from build123d import *

# Parameters (mm, degrees)
SKETCH1_W           = 40
SKETCH1_H           = 8
SKETCH1_R           = 0.75
BOSS_EXTRUDE1_DEPTH = 3
SKETCH2_W           = 19
SKETCH2_H           = 8
BOSS_EXTRUDE2_DEPTH = 15
SKETCH3_W           = 12.3
SKETCH3_H           = 29.8
CUT_EXTRUDE1_DEPTH  = 8
FILLET1_R           = 1


with BuildPart() as part:
    # Sketch1 → Boss-Extrude1 (new body)
    with BuildSketch(Plane.XY):
        Rectangle(SKETCH1_W, SKETCH1_H)
        with Locations((-14.5, 0)):
            Circle(SKETCH1_R, mode=Mode.SUBTRACT)
        with Locations((14.5, 0)):
            Circle(SKETCH1_R, mode=Mode.SUBTRACT)
    extrude(amount=BOSS_EXTRUDE1_DEPTH)

    # Sketch2 → Boss-Extrude2 (add)
    with BuildSketch(Plane.XY.offset(3)):
        Rectangle(SKETCH2_W, SKETCH2_H)
    extrude(amount=BOSS_EXTRUDE2_DEPTH)

    # Sketch3 → Cut-Extrude1 (cut)
    with BuildSketch(Plane.XZ.offset(4)):
        Rectangle(SKETCH3_W, SKETCH3_H)
    extrude(amount=-CUT_EXTRUDE1_DEPTH, mode=Mode.SUBTRACT)

    # Fillet1
    fillet1_edges = [part.edges().sort_by_distance(p)[0] for p in [
        (-9.5, 0, 3),
        (9.5, 0, 3),
        (-9.5, 0, 18),
        (9.5, 0, 18),
    ]]
    fillet(fillet1_edges, radius=FILLET1_R)


solid = part.part
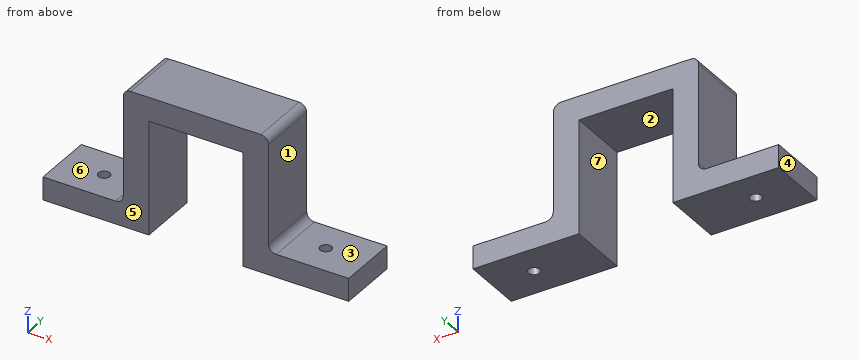
Input: part model. Units: mm. Frame: model coordinates. Face numbers are marked on the shaded views. A direction names the side the tool comes from. Coordinates: 2 decimals unless noted, no trailing zeros. Loops run counter-clockwise (first coordinate to the right, second up) from the corner with the lowest first, then second, coordinate; pieces in that order, holes last. Notation, with made-up numbers: (67.5, 19.5) -> (123.5, 19.5) arc R18 cw to (123.5, 26.5) -> close; hole circle Ø9 at (80.5, 38). An arc over 180 degrees is marked (long way). Write item = value, one per line. Start each with the question number.
Item 1: Material intervals for line 1 (X direction, y = -2.25, z = 14.5); line 2 (Y direction, x = -14.5, z = 2.05); line 3 (X direction, y = 1.5, z = 2), sorted ascending.
Item 2: First-contact query: P1, Ø1.4, axis at x = -14.5, y = 0, coming from the -Z side; P2, Ø4, axis at y = 1.5, z = 10.5, coming from the -X side; P3, Ø2.5, axis at x = 17.5, y = -2, coming from the +Z side; P4, Ø2, axis at x = 2, y = 0, coming from the -Z side. Flat tips, straight axial feed; report the tip coordinate or a pass-through.
Item 3: Cut plane A-A, the plane z = 6.5. Return loops of the section in (x, y).
Item 4: Cut plane D-D, the plane y = 2. Return loops of the section in (x, z), plus the area to 3 significant figures.
Item 5: Cut plane B-B, the plane x = 14.5. Return loops of the section in (y, z), plus the area to 3 significant figures.
Item 6: Reachability of the marked faces 5, 6 and 7 from +Z, -Z, +X, -X, +Y, -Y: full face, straight path, thin tool, end or side. Return the list, or none.
Item 7: Mould query, pull axis X, two halves, no side actions, for the marked faces 1, 2, 3 and 4. Classes: pulls with the +X half, pulls with the -X half, needs draft (parallel to the pull), parting line crosses it, or undercut.
Item 8: Cut plane C-C, the plane y = 0. Return loops of the section in (x, z), plus the area to 3 significant figures.
Ans:
q1.line_1 = -9.5 to -6.15, 6.15 to 9.5
q1.line_2 = -4 to -0.75, 0.75 to 4
q1.line_3 = -20 to -6.15, 6.15 to 20
q2.P1 = through
q2.P2 = -9.5
q2.P3 = 3
q2.P4 = 14.9
q3.outline = (-9.5, -4) -> (-6.15, -4) -> (-6.15, 4) -> (-9.5, 4) -> close; (6.15, -4) -> (9.5, -4) -> (9.5, 4) -> (6.15, 4) -> close
q4.outline = (-20, 0) -> (-6.15, 0) -> (-6.15, 14.9) -> (6.15, 14.9) -> (6.15, 0) -> (20, 0) -> (20, 3) -> (10.5, 3) arc R1 cw to (9.5, 4) -> (9.5, 17) arc R1 ccw to (8.5, 18) -> (-8.5, 18) arc R1 ccw to (-9.5, 17) -> (-9.5, 4) arc R1 cw to (-10.5, 3) -> (-20, 3) -> close
q4.area = 222 mm²
q5.outline = (-4, 0) -> (-0.75, 0) -> (-0.75, 3) -> (-4, 3) -> close; (0.75, 0) -> (4, 0) -> (4, 3) -> (0.75, 3) -> close
q5.area = 19.5 mm²
q6.face_5 = +Z, -Z, +X, -X, -Y
q6.face_6 = +Z, -X, +Y, -Y
q6.face_7 = -Z, +Y, -Y
q7.face_1 = pulls with the +X half
q7.face_2 = undercut
q7.face_3 = needs draft
q7.face_4 = pulls with the -X half
q8.outline = (-20, 0) -> (-15.25, 0) -> (-15.25, 3) -> (-20, 3) -> close; (-13.75, 0) -> (-6.15, 0) -> (-6.15, 14.9) -> (6.15, 14.9) -> (6.15, 0) -> (13.75, 0) -> (13.75, 3) -> (10.5, 3) arc R1 cw to (9.5, 4) -> (9.5, 17) arc R1 ccw to (8.5, 18) -> (-8.5, 18) arc R1 ccw to (-9.5, 17) -> (-9.5, 4) arc R1 cw to (-10.5, 3) -> (-13.75, 3) -> close; (15.25, 0) -> (20, 0) -> (20, 3) -> (15.25, 3) -> close
q8.area = 213 mm²
